from build123d import *

# Parameters (mm, degrees)
F2_R     = 5.25
F3_DEPTH = 22
F5_START = 22
F4_R     = 11
F5_DEPTH = 10


with BuildPart() as f3:
    # F2 (on Top) → F3 (new body)
    with BuildSketch(Plane.XY):
        Circle(F2_R)
    extrude(amount=F3_DEPTH)

    # F4 (on Top) → F5 (join)
    with BuildSketch(Plane.XY.offset(F5_START)):
        Circle(F4_R)
    extrude(amount=F5_DEPTH)

    # F6 (on Front) → F7 (revolve)
    with BuildSketch(Plane.XZ):
        Polygon((0, 11), (0, 22), (-11, 22), align=None)
    revolve(axis=Axis((0, 0, 16.5), (0, 0, 1)))


solid = f3.part
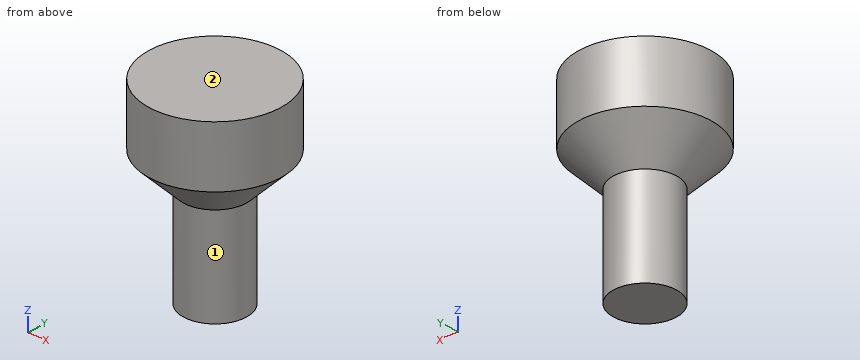
For this review, take the finished solid that the model builds, in its own axes (mm). Face numbers are marked on the shaded views. A direction names the side the tool comes from. Give positions to 0.01 mm unless a question says otherwise; leave off trailing zeros. Order: outer loops, then holes, each group sorted by start corner. A loop starts at its lowest first (then second) coordinate and runs counter-clockwise, first axis right, second up. Notation, with made-up numbers: M 74.25,-31 L 107.25,-31 A31 cw 107.25,-3 Z; hole C 77,-28 d2. An arc over 180 degrees is marked long. Answer in a Markdown table with one row per item. Add a question column.
(1) Wall thickness on probe 1 along Y at (x, z) = (0, 8); probe 2 along Y at (x, z) = (-2.5, 5); probe 3 along Z at (x, y) = (-2.75, 9.25): over which ranges is each line inside the solid? List them lowest first. Write a range as [from, to].
(2) Consider section A-A on x = 0. State the section outline as (y, z) points, and give its area (3 significant figures).
(3) For pin 1 (1.5 mm diameter, centred on x = 8.5, z = 27, fed in from +Y); pin 2 (2 mm diameter, centred on y = 2, z = 23, fed in from +X); pin 3 (1.5 mm diameter, centred on x = -7.5, z = 27, fed in from -Y), all flat-tipped, find the tip position at first contact; note any pin that passes through.
(4) Consider section D-D on z = 26.5. State the section outline as (x, y) points, and give its area (3 significant figures).
(5) For the marked faces 1 and 2, list the 3-axis set-ups (+Z, -Z, +X, -X, +Y, -Y) from which the entire face can be reached by the end or side of a thin tool; tool diameter is ignored.
(6) Consider section C-C on z = 4.5. State the section outline as (x, y) points, and give its area (3 significant figures).
Evaluation:
| question | item | result |
|---|---|---|
| 1 | probe 1 | y = [-5.25, 5.25] |
| 1 | probe 2 | y = [-4.62, 4.62] |
| 1 | probe 3 | z = [20.65, 32] |
| 2 | outline | M -11,22 L -5.25,16.25 L -5.25,0 L 5.25,0 L 5.25,16.25 L 11,22 L 11,32 L -11,32 Z |
| 2 | area | 484 mm^2 |
| 3 | pin 1 | stops at y = 7.81 |
| 3 | pin 2 | stops at x = 10.95 |
| 3 | pin 3 | stops at y = -8.69 |
| 4 | outline | C 0,0 d22 |
| 4 | area | 380 mm^2 |
| 5 | face 1 | -Z |
| 5 | face 2 | +Z, +X, -X, +Y, -Y |
| 6 | outline | C 0,0 d10.5 |
| 6 | area | 86.6 mm^2 |
